```python
from build123d import *

# Parameters (mm, degrees)
ESQUISSE1_W             = 34
ESQUISSE1_H             = 42
BOSS_EXTRU_1_DEPTH      = 7
ESQUISSE2_W             = 31
ESQUISSE2_H             = 28
ENL_V_MAT_EXTRU_1_DEPTH = 4
ESQUISSE3_R             = 2.5
ENL_V_MAT_EXTRU_2_DEPTH = 55.488530903
ESQUISSE4_R             = 7
ESQUISSE4_R_2           = 1.5
ENL_V_MAT_EXTRU_3_DEPTH = 4
ESQUISSE5_R             = 1.5
ENL_V_MAT_EXTRU_4_DEPTH = 4
CHANFREIN2_SIZE         = 0.25


with BuildPart() as part:
    # Esquisse1 → Boss.-Extru.1 (new body)
    with BuildSketch(Plane.XY):
        with Locations((17, 21)):
            Rectangle(ESQUISSE1_W, ESQUISSE1_H)
    extrude(amount=BOSS_EXTRU_1_DEPTH)

    # Esquisse2 → Enlèv. mat.-Extru.1 (cut)
    with BuildSketch(Plane.XY.offset(7)):
        with Locations((15.5, 21)):
            Rectangle(ESQUISSE2_W, ESQUISSE2_H)
    extrude(amount=-ENL_V_MAT_EXTRU_1_DEPTH, mode=Mode.SUBTRACT)

    # Esquisse3 → Enlèv. mat.-Extru.2 (cut, through all)
    with BuildSketch(Plane.ZY):
        with Locations((3.5, 38.5)):
            Circle(ESQUISSE3_R)
        with Locations((3.5, 3.5)):
            Circle(ESQUISSE3_R)
    extrude(amount=-ENL_V_MAT_EXTRU_2_DEPTH, mode=Mode.SUBTRACT)

    # Esquisse4 → Enlèv. mat.-Extru.3 (cut)
    with BuildSketch(Plane.XY.offset(3)):
        with Locations((15.5, 21)):
            Circle(ESQUISSE4_R)
        with Locations((15.5, 31)):
            Circle(ESQUISSE4_R_2)
        with Locations((15.5, 11)):
            Circle(ESQUISSE4_R_2)
        with Locations((25.5, 21)):
            Circle(ESQUISSE4_R_2)
        with Locations((5.5, 21)):
            Circle(ESQUISSE4_R_2)
    extrude(amount=-ENL_V_MAT_EXTRU_3_DEPTH, mode=Mode.SUBTRACT)

    # Esquisse5 → Enlèv. mat.-Extru.4 (cut)
    with BuildSketch(Plane(origin=(34, 0, 0), x_dir=(0, 0, -1), z_dir=(1, 0, 0))):
        with Locations(Location((-5, 21, 0), (0, 0, 90))):
            Circle(ESQUISSE5_R)
    extrude(amount=-ENL_V_MAT_EXTRU_4_DEPTH, mode=Mode.SUBTRACT)

    # Chanfrein2
    chanfrein2_edges = [part.edges().sort_by_distance(p)[0] for p in [
        (34, 21, 7),
        (17, 42, 7),
        (0, 3.5, 7),
        (0, 21, 3),
        (0, 7, 5),
        (15.5, 35, 3),
        (0, 35, 5),
        (31, 21, 3),
        (31, 35, 5),
        (15.5, 7, 3),
        (31, 7, 5),
        (15.5, 7, 7),
        (31, 21, 7),
        (15.5, 35, 7),
        (34, 38.5, 1),
        (0, 38.5, 1),
        (34, 3.5, 1),
        (0, 3.5, 1),
        (0, 38.5, 7),
        (14, 31, 0),
        (14, 31, 3),
        (17, 42, 0),
        (14, 11, 0),
        (14, 11, 3),
        (24, 21, 0),
        (24, 21, 3),
        (34, 21, 0),
        (4, 21, 0),
        (4, 21, 3),
        (8.5, 21, 0),
        (8.5, 21, 3),
        (17, 0, 0),
        (0, 21, 0),
        (31, 19.5, 5),
        (34, 19.5, 5),
        (17, 0, 7),
        (0, 42, 3.5),
        (34, 42, 3.5),
        (34, 0, 3.5),
        (0, 0, 3.5),
    ]]
    chamfer(chanfrein2_edges, length=CHANFREIN2_SIZE - 0.0001)  # a hair under: the kernel refuses the full size


solid = part.part
```
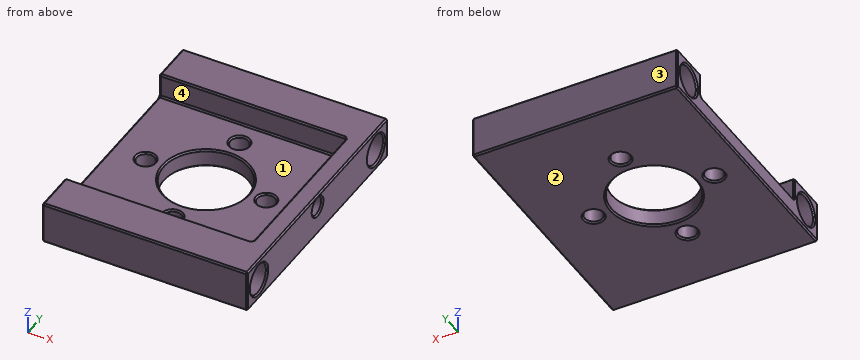
The listing builds one solid part. Answer for the finished solid, in the listing's coordinates (mm). Face numbers are marked on the shaded views. Round coordinates to 2 decimals unless told otherwise and drop trailing zeros. Loops run counter-clockwise (first coordinate to the right, second up) from the corner with the lowest first, then second, coordinate; pieces in that order, holes last.
Q1. Given pin 1 Ø1.8 at (x, y) = (15.5, 11) entering from +Z; pin 2 Ø1 at (x, y) = (23, 33.5) entering from +Z; pin 3 Ø2 at (y, z) = (21.5, 6) entering from -X, each flat-ended and moving along its own axis, determine where each tip first touches the part or whether it passes through.
Q2. Section A-A, the plane x = 5.5 is taken. Determine the outline of the cut face in (y, z).
Q3. Find the intervals of material crossed by line 1 (Y direction, x = 23.5, z = 3.5); line 2 (Y direction, x = 28.5, z = 2.5); line 3 (Y direction, x = 25.5, z = 1.4), in increasing order.
Q4. For a pull along Y with two mould halves and no side action, classify the marked faces 1, 2, 3 and 4 as released by +Y, released by -Y, zero draft, split by the parting line, or undercut.
Q5. Section B-B, the plane y = 31 is taken. Determine the outline of the cut face in (x, z), then the cut area to 3 significant figures.
Q6. Section D-D, the plane y = 3.5 is taken. Determine the outline of the cut face in (x, z).
Q7. Section C-C, the plane x = 15.5 is taken. Count the separate pieces of the cut face and the enclosed holes in it, then the cut area to 3 significant figures.
Completed:
1. pin 1: passes through
1. pin 2: stops at z = 3
1. pin 3: stops at x = 31
2. outline: (0, 0.25) - (0.25, 0) - (19.25, 0) - (19.5, 0.25) - (19.5, 2.75) - (19.25, 3) - (7.25, 3) - (7, 3.25) - (7, 6.75) - (6.75, 7) - (0.25, 7) - (0, 6.75) - close; (22.5, 0.25) - (22.75, 0) - (41.75, 0) - (42, 0.25) - (42, 6.75) - (41.75, 7) - (35.25, 7) - (35, 6.75) - (35, 3.25) - (34.75, 3) - (22.75, 3) - (22.5, 2.75) - close; hole circle Ø5 at (3.5, 3.5); hole circle Ø5 at (38.5, 3.5)
3. line 1: y = 0 to 1, 6 to 7, 35 to 36, 41 to 42
3. line 2: y = 0 to 1.21, 5.79 to 36.21, 40.79 to 42
3. line 3: y = 0 to 2.14, 4.86 to 19.5, 22.5 to 37.14, 39.86 to 42
4. face 1: undercut
4. face 2: zero draft
4. face 3: released by +Y
4. face 4: undercut
5. outline: (0, 0.25) - (0.25, 0) - (13.75, 0) - (14, 0.25) - (14, 2.75) - (13.75, 3) - (0.25, 3) - (0, 2.75) - close; (17, 0.25) - (17.25, 0) - (33.75, 0) - (34, 0.25) - (34, 6.75) - (33.75, 7) - (31.25, 7) - (31, 6.75) - (31, 3.25) - (30.75, 3) - (17.25, 3) - (17, 2.75) - close
5. area: 105 mm2
6. outline: (0, 0.25) - (0.25, 0) - (33.75, 0) - (34, 0.25) - (34, 0.75) - (33.75, 1) - (0.25, 1) - (0, 0.75) - close; (0, 6.25) - (0.25, 6) - (33.75, 6) - (34, 6.25) - (34, 6.75) - (33.75, 7) - (0.25, 7) - (0, 6.75) - close
7. separate pieces: 4
7. enclosed holes: 2
7. area: 82.2 mm2
